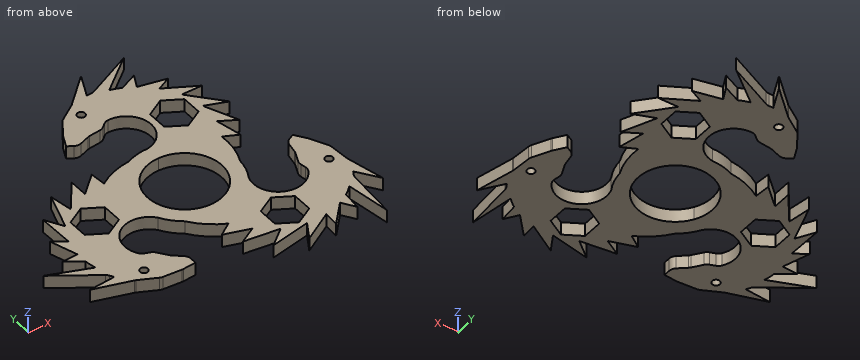
```python
from build123d import *

# Parameters (mm, degrees)
F0_R     = 1.5
F1_DEPTH = 5
F3_COUNT = 3


# Not quite as in the source:
# - a feature names something its author has since deleted; it is built from what else it names


with BuildPart() as f1:
    # F0 (on Top) → F1 (new body)
    with BuildSketch(Plane.XY):
        with BuildLine():
            ThreePointArc((-1.7478732612, 39.5149783142), (8.1392001596, 30.7821912097), (0, 20.4009960858))
            Line((0, 20.4009960858), (0, 14.4152096754))
            ThreePointArc((0, 14.4152096754), (12.4839377798, 7.2076048377), (12.4839377798, -7.2076048377))
            Line((12.4839377798, -7.2076048377), (17.6677808728, -10.2004980429))
            ThreePointArc((17.6677808728, -10.2004980429), (19.4452285789, -6.171201407), (20.3165472355, -1.8543326892))
            ThreePointArc((20.3165472355, -1.8543326892), (22.4085751719, 4.7991946551), (22.7576271971, 11.7651238603))
            Line((22.7576271971, 11.7651238603), (28.2481051981, 9.1530177742))
            Line((28.2481051981, 9.1530177742), (26.0387565941, 19.0982837094))
            Line((26.0387565941, 19.0982837094), (32.3511809111, 15.4654439539))
            Line((32.3511809111, 15.4654439539), (26.9242947963, 28.0441137764))
            Line((26.9242947963, 28.0441137764), (35.1917743683, 24.9340832233))
            Line((35.1917743683, 24.9340832233), (24.8427105993, 36.6120710969))
            Line((24.8427105993, 36.6120710969), (32.6668024063, 36.6120710969))
            Line((32.6668024063, 36.6120710969), (20.8077298225, 43.1800760308))
            Line((20.8077298225, 43.1800760308), (26.0387565941, 45.7650870085))
            Line((26.0387565941, 45.7650870085), (15.485866915, 48.02231204))
            Line((15.485866915, 48.02231204), (18.1482266635, 53.3400028944))
            Line((18.1482266635, 53.3400028944), (11.520179105, 50.2734731867))
            ThreePointArc((11.520179105, 50.2734731867), (9.4992839441, 51.1021592503), (7.4171009474, 51.7618954182))
            Line((7.4171009474, 51.7618954182), (20.6731967628, 62.493018806))
            Line((20.6731967628, 62.493018806), (2.9851620813, 53.9539658583))
            ThreePointArc((2.9851620813, 53.9539658583), (2.3498823759, 53.7311579429), (1.6809146705, 53.6556206644))
            Line((1.6809146705, 53.6556206644), (0, 53.6556206644))
            Line((0, 53.6556206644), (4.2608887888, 62.8086403012))
            Line((4.2608887888, 62.8086403012), (-6.6135251858, 52.5556231266))
            ThreePointArc((-6.6135251858, 52.5556231266), (-6.7917072446, 52.4004137483), (-6.9815525166, 52.2597099106))
            Line((-6.9815525166, 52.2597099106), (-13.2472028108, 47.9876733272))
            ThreePointArc((-13.2472028108, 47.9876733272), (-13.6895314092, 47.6192351761), (-14.0533422232, 47.1730928761))
            Line((-14.0533422232, 47.1730928761), (-18.0220315222, 41.2200618552))
            ThreePointArc((-18.0220315222, 41.2200618552), (-18.1407171431, 41.0265497088), (-18.2444304369, 40.824617096))
            Line((-18.2444304369, 40.824617096), (-20.3575752676, 36.2964496017))
            Line((-20.3575752676, 36.2964496017), (-18.2173253559, 35.0123005809))
            ThreePointArc((-18.2173253559, 35.0123005809), (-16.9608718875, 34.5985427406), (-15.6486105692, 34.7653992696))
            Line((-15.6486105692, 34.7653992696), (-11.8852458251, 36.1338942554))
            ThreePointArc((-11.8852458251, 36.1338942554), (-11.5431146027, 36.2357083507), (-11.1913122519, 36.2961648589))
            Line((-11.1913122519, 36.2961648589), (-6.7715043443, 36.7872549082))
            ThreePointArc((-6.7715043443, 36.7872549082), (-5.920047927, 37.0118969078), (-5.1704976221, 37.4740834492))
            Line((-5.1704976221, 37.4740834492), (-3.5822876233, 38.8113983631))
            ThreePointArc((-3.5822876233, 38.8113983631), (-2.7243104061, 39.3176161279), (-1.7478732612, 39.5149783142))
        make_face()
        with Locations((-7.1445683185, 46.6340765733)):
            Circle(F0_R, mode=Mode.SUBTRACT)
        Polygon((10.8037195943, 34.1769884273), (17.5, 38.0430877221), (24.1962804057, 34.1769884273), (24.1962804057, 26.4447898377), (17.5, 22.5786905429), (10.8037195943, 26.4447898377), align=None, mode=Mode.SUBTRACT)
    extrude(amount=F1_DEPTH)

    # F3: F1 ×3 about axis
    f3_axis = Axis((0, 0, 21.8280367553), (0, 0, 1))


with BuildPart() as f1_1:
    add(f1.part)
    for i in range(1, F3_COUNT):
        add(f1.part.rotate(f3_axis, i * 360 / F3_COUNT))


solid = f1_1.part
```
The listing builds one solid part. Answer for the finished solid, in the listing's coordinates (mm). Round coordinates to 2 decimals unless told otherwise and drop trailing zeros. Loops run counter-clockwise (first coordinate to the right, second up) from the corner with the lowest first, then second, coordinate; pieces in that order, holes last. Notation, with made-up numbers: (83.5, 5.25) - (98.5, 5.25) arc R24 ccw to (98.5, 29.25) - close; hole circle Ø6 at (27.25, -13.5). An arc over 180 degrees is marked (long way). Return JSON: item names as keys, results as strings. Group by question number.
1. Each of these flat-tipped pins is pushed along its axis until it touches: P1, Ø2, axis at x = 36, z = 1, coming from the -Y side; P2, Ø5, axis at x = 43.96, y = -17.13, coming from the +Z side; P3, Ø2.5, axis at x = -7.14, y = 46.63, coming from the -Z side; P4, Ø1.5, axis at x = -31, z = 3.5, coming from the +Y side. Where does it stop, or does it pass through?
2. The part is cut by section A-A on x = 31. Determine the outline of the cut face in (y, z).
3. The part is cut by section B-B on y = 55.5. Determine the outline of the cut face in (x, z), then the cut area to 3 significant figures.
4. Consider probe 1 along X at (y, z) = (-22, 0.3); probe 2 along X at (y, z) = (-32.5, 2.25); probe 3 along X at (y, z) = (7.5, 0.95). Determine where each line is inside the solid, lowest interval first.
5. The part is cut by section C-C on z = 2.9. State how many separate pieces and enclosed holes the cut face has, then the cut area to 3 significant figures.
Resolved:
{
 "1": {"P1": "stops at y = -42.21", "P2": "stops at z = 5", "P3": "passes through", "P4": "stops at y = 19.37"},
 "2": {"outline": "(-40.57, 0) - (-22.27, 0) - (-22.27, 5) - (-40.57, 5) - close; (16.24, 0) - (18.6, 0) - (18.6, 5) - (16.24, 5) - close; (26.51, 0) - (29.66, 0) - (29.66, 5) - (26.51, 5) - close; (36.61, 0) - (37.54, 0) - (37.54, 5) - (36.61, 5) - close"},
 "3": {"outline": "(-3.49, 0) - (0.86, 0) - (0.86, 5) - (-3.49, 5) - close; (6.19, 0) - (12.03, 0) - (12.03, 5) - (6.19, 5) - close", "area": "51.0 mm²"},
 "4": {"probe 1": "x = -51.73 to -32.71, -6.82 to 21.75, 31.49 to 49.16", "probe 2": "x = -41.09 to -21.3, 2.83 to 10.8, 24.2 to 40.92, 41.15 to 45.02, 50.44 to 51.65", "probe 3": "x = -48 to -46.61, -42.7 to -35.4, -34.6 to -12.31, 12.31 to 22.76"},
 "5": {"separate pieces": "1", "enclosed holes": "7", "area": "3,780 mm²"}
}
